Input: part model. Units: mm. Frame: model coordinates. Face numbers are marked on the shaded views. A direction names the side the tool comes from. Give positions to 0.01 mm unless a question says otherwise; leave off trailing zeros. Loops run counter-clockwise (first coordinate to the right, second up) from the corner with the lowest first, then second, coordinate; pieces in that order, holes last. Notation, with made-up numbers: (82.5, 58) - (98.5, 58) arc R22 ccw to (98.5, 83) - close; hole circle Ø3 at (-37.5, 22.25). An arc over 180 degrees is marked (long way). Answer as a JSON object with one key per item and string values. Group by question number.
(1) Section query D-D (z = 6.5). Return loops of the section in (x, y) (3 decimals), plus the area to 3 significant figures.
(2) Section query A-A (x = -15). Return loops of the section in (y, z).
(3) Section query C-C (y = -45.5). Return loops of the section in (x, z) (3 decimals), plus the area to 3 significant figures.
(4) Material intervals for L1, parallel to Y at x = -5.5, z = 2.75; L2, parallel to Z at x = -26, y = -14; L3, parallel to X at y = -24, z = 7 (3 decimals), sorted ascending.
(5) Pin query (flat end, axial travel): P1, Ø6, axis at y = -38.1, z = 14.605, coming from the +X side (3 decimals); P2, Ø3, axis at x = -28, y = -33, coming from the +Z side. Return the tip coordinate at first contact, or that it passes through.
(6) Access query for the marked faces 1 and 2. Directions: +Z, -Z, +X, -X, +Y, -Y. A direction counts if a zero-diameter tool reaches every point of the face in a straight line with its end or side. Return the directions, or none.
(7) Section query B-B (y = -12.7). Return loops of the section in (x, z) (3 decimals).
```python
from build123d import *

# Parameters (mm, degrees)
F1_DEPTH = 50.8
F2_W     = 21.9075
F2_H     = 3.2512
F3_DEPTH = 25.4
F4_R     = 2.286
F5_DEPTH = 25.4


with BuildPart() as f1:
    # F0 (on Front) → F1 (new body)
    with BuildSketch(Plane.XZ):
        Polygon((-34.925, 0), (0, 0), (0, 5.08), (-29.845, 5.08), (-29.845, 19.05), (-34.925, 19.05), align=None)
    extrude(amount=F1_DEPTH)

    # F2 (on face) → F3 (cut)
    with BuildSketch(Plane.XY.offset(5.08)):
        with Locations((-15.71625, -41.275)):
            Rectangle(F2_W, F2_H)
        with Locations((-15.71625, -9.525)):
            Rectangle(F2_W, F2_H)
    extrude(amount=-F3_DEPTH, mode=Mode.SUBTRACT)

    # F4 (on face) → F5 (cut)
    with BuildSketch(Plane.YZ.offset(-29.845)):
        with Locations((-38.1, 14.605)):
            Circle(F4_R)
        with Locations((-12.7, 14.605)):
            Circle(F4_R)
    extrude(amount=-F5_DEPTH, mode=Mode.SUBTRACT)


solid = f1.part
```
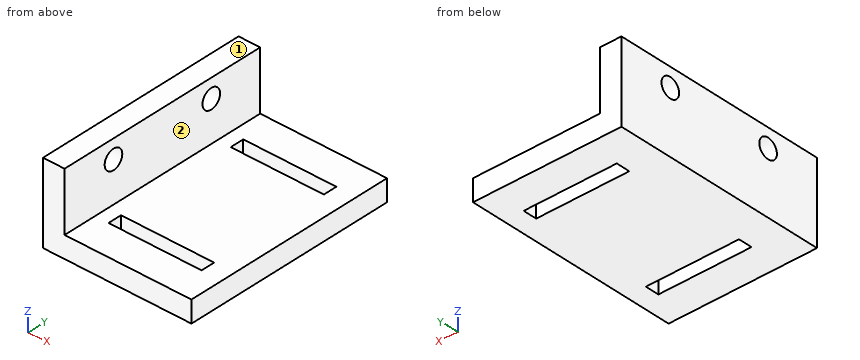
Recorded:
{
 "1": {"outline": "(-34.925, -50.8) - (-29.845, -50.8) - (-29.845, 0) - (-34.925, 0) - close", "area": "258 mm^2"},
 "2": {"outline": "(-50.8, 0) - (-42.9, 0) - (-42.9, 5.08) - (-50.8, 5.08) - close; (-39.65, 0) - (-11.15, 0) - (-11.15, 5.08) - (-39.65, 5.08) - close; (-7.9, 0) - (0, 0) - (0, 5.08) - (-7.9, 5.08) - close"},
 "3": {"outline": "(-34.925, 0) - (0, 0) - (0, 5.08) - (-29.845, 5.08) - (-29.845, 19.05) - (-34.925, 19.05) - close", "area": "248 mm^2"},
 "4": {"L1": "y = -50.8 to -42.9, -39.65 to -11.15, -7.9 to 0", "L2": "z = 0 to 5.08", "L3": "x = -34.925 to -29.845"},
 "5": {"P1": "stops at x = -29.845", "P2": "stops at z = 5.08"},
 "6": {"face 1": "+Z, +X, -X, +Y, -Y", "face 2": "+Z, +X, +Y, -Y"},
 "7": {"outline": "(-34.925, 0) - (0, 0) - (0, 5.08) - (-29.845, 5.08) - (-29.845, 12.319) - (-34.925, 12.319) - close; (-34.925, 16.891) - (-29.845, 16.891) - (-29.845, 19.05) - (-34.925, 19.05) - close"}
}
